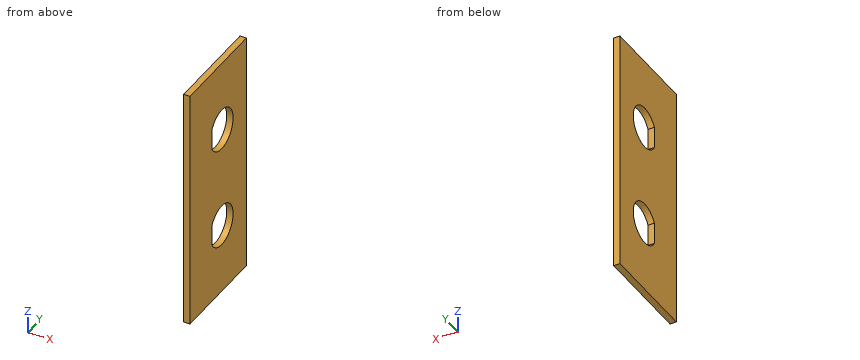
from build123d import *

# Parameters (mm, degrees)
SKETCH1_W           = 203.2
SKETCH1_H           = 120.65
BOSS_EXTRUDE1_DEPTH = 50.8
SKETCH2_W           = 196.85
SKETCH2_H           = 114.3
CUT_EXTRUDE1_DEPTH  = 51.8
SKETCH4_W           = 203.2
SKETCH4_H           = 120.65
SKETCH4_W_2         = 196.85
SKETCH4_H_2         = 114.3
BOSS_EXTRUDE2_DEPTH = 6.35
CUT_EXTRUDE5_DEPTH  = 121.65
CUT_EXTRUDE6_REACH  = 205.2
CUT_EXTRUDE7_REACH  = 205.2
SKETCH13_R          = 12.55395
SKETCH14_W          = 200.025
SKETCH14_H          = 120.65
CUT_EXTRUDE8_DEPTH  = 51.8


with BuildPart() as part:
    # Sketch1 → Boss-Extrude1 (new body)
    with BuildSketch(Plane(origin=(0, 0, 0), x_dir=(1, 0, 0), z_dir=(0, 1, 0))):
        Rectangle(SKETCH1_W, SKETCH1_H)
    extrude(amount=BOSS_EXTRUDE1_DEPTH)

    # Sketch2 → Cut-Extrude1 (cut, through all)
    with BuildSketch(Plane(origin=(0, 50.8, 0), x_dir=(1, 0, 0), z_dir=(0, 1, 0))):
        Rectangle(SKETCH2_W, SKETCH2_H)
    extrude(amount=-CUT_EXTRUDE1_DEPTH, mode=Mode.SUBTRACT)

    # Sketch4 → Boss-Extrude2 (add)
    with BuildSketch(Plane(origin=(0, 50.8, 0), x_dir=(1, 0, 0), z_dir=(0, 1, 0))):
        Rectangle(SKETCH4_W, SKETCH4_H)
        Rectangle(SKETCH4_W_2, SKETCH4_H_2, mode=Mode.SUBTRACT)
    extrude(amount=-BOSS_EXTRUDE2_DEPTH)

    # Sketch10 → Cut-Extrude5 (cut, through all)
    with BuildSketch(Plane.XY.offset(60.325)):
        with BuildLine():
            ThreePointArc((-65.9511, 22.225), (-81.206975571, 31.167602912), (-81.556705839, 13.4874))
            Line((-81.556705839, 13.4874), (-70.843294161, 13.4874))
            ThreePointArc((-70.843294161, 13.4874), (-67.257397088, 17.218024429), (-65.9511, 22.225))
        make_face()
        with BuildLine():
            ThreePointArc((-15.1511, 22.225), (-30.406975571, 31.167602912), (-30.756705839, 13.4874))
            Line((-30.756705839, 13.4874), (-20.043294161, 13.4874))
            ThreePointArc((-20.043294161, 13.4874), (-16.457397088, 17.218024429), (-15.1511, 22.225))
        make_face()
        with BuildLine():
            ThreePointArc((35.6489, 22.225), (20.393024429, 31.167602912), (20.043294161, 13.4874))
            Line((20.043294161, 13.4874), (30.756705839, 13.4874))
            ThreePointArc((30.756705839, 13.4874), (34.342602912, 17.218024429), (35.6489, 22.225))
        make_face()
        with BuildLine():
            Line((70.843294161, 13.4874), (81.556705839, 13.4874))
            ThreePointArc((81.556705839, 13.4874), (85.142602912, 17.218024429), (86.4489, 22.225))
            ThreePointArc((86.4489, 22.225), (71.193024429, 31.167602912), (70.843294161, 13.4874))
        make_face()
    extrude(amount=-CUT_EXTRUDE5_DEPTH, mode=Mode.SUBTRACT)

    # Sketch12 → Cut-Extrude6 (cut, up to next)
    with BuildSketch(Plane(origin=(101.6, 0, 0), x_dir=(0, 0, -1), z_dir=(1, 0, 0)), mode=Mode.PRIVATE) as cut_extrude6_sk1:
        with BuildLine():
            ThreePointArc((-20.043294161, 19.8374), (-25.4, 38.8239), (-30.756705839, 19.8374))
            Line((-30.756705839, 19.8374), (-20.043294161, 19.8374))
        make_face()
    cut_extrude6_tool1 = extrude(cut_extrude6_sk1.sketch, amount=-CUT_EXTRUDE6_REACH, mode=Mode.PRIVATE) & part.part
    add(cut_extrude6_tool1.solids().sort_by_distance((101.6, 28.896198, 25.4))[0], mode=Mode.SUBTRACT)
    # Sketch12 → Cut-Extrude6 (cut, up to next)
    with BuildSketch(Plane(origin=(101.6, 0, 0), x_dir=(0, 0, -1), z_dir=(1, 0, 0)), mode=Mode.PRIVATE) as cut_extrude6_sk2:
        with BuildLine():
            ThreePointArc((30.756705839, 19.8374), (25.4, 38.8239), (20.043294161, 19.8374))
            Line((20.043294161, 19.8374), (30.756705839, 19.8374))
        make_face()
    cut_extrude6_tool2 = extrude(cut_extrude6_sk2.sketch, amount=-CUT_EXTRUDE6_REACH, mode=Mode.PRIVATE) & part.part
    add(cut_extrude6_tool2.solids().sort_by_distance((101.6, 28.896198, -25.4))[0], mode=Mode.SUBTRACT)

    # Sketch13 → Cut-Extrude7 (cut, up to next)
    with BuildSketch(Plane.ZY.offset(101.6), mode=Mode.PRIVATE) as cut_extrude7_sk1:
        with Locations((15.875, 28.575)):
            Circle(SKETCH13_R)
    cut_extrude7_tool1 = extrude(cut_extrude7_sk1.sketch, amount=-CUT_EXTRUDE7_REACH, mode=Mode.PRIVATE) & part.part
    add(cut_extrude7_tool1.solids().sort_by_distance((-101.6, 28.575, 15.875))[0], mode=Mode.SUBTRACT)

    # Sketch14 → Cut-Extrude8 (cut, through all)
    with BuildSketch(Plane(origin=(0, 50.8, 0), x_dir=(1, 0, 0), z_dir=(0, 1, 0))):
        with Locations((-1.5875, 0)):
            Rectangle(SKETCH14_W, SKETCH14_H)
    extrude(amount=-CUT_EXTRUDE8_DEPTH, mode=Mode.SUBTRACT)


solid = part.part
CAD build for the part. Positions are in the model's coordinates, mm. Round coordinates to 2 decimals unless told otherwise and drop trailing zeros. Write each loop counter-clockwise with the first axis right and the second up, starting at its lowest first coordinate (ties: lowest second). Pieces come first, ordered by that corner, then holes. Notation, with made-up numbers: M 51,21 L 94,21 A13 ccw 94,36 Z; hole C -24,42.5 d4. An arc over 180 degrees is marked long. Put each result on its own line as item: value. Start each with the question number.
1) Saw through at B-B, the plane y = 28. Write the cut outline in (x, z) (3 decimals).
2) Saw through at C-C, the plane x = 100.45. Write the cut outline in (y, z) (3 decimals).
3) Saw through at A-A, the plane z = 25.4. Write the cut outline in (x, y) (3 decimals), and give its area (3 significant figures).
4) Drill centre lines: probe 1 along Z at (x, y) = (100.4, 37) (3 decimals); probe 2 along Z at (x, y) = (99.65, 21) (3 decimals); probe 3 along Y at (x, z) = (99.9, -25.4). Where is each one in solid material? Low to high. Write a range as [from, to].
5) Pin check, flat tip, straight feed: pin 1 Ø23.5 at (y, z) = (28.575, -25.4) entering from +X. Stop position of the tip, or through.
Resolved:
1. outline: M 98.425,-60.325 L 101.6,-60.325 L 101.6,-35.633 L 98.425,-35.633 Z; M 98.425,-15.167 L 101.6,-15.167 L 101.6,15.167 L 98.425,15.167 Z; M 98.425,35.633 L 101.6,35.633 L 101.6,60.325 L 98.425,60.325 Z
2. outline: M 0,-60.325 L 50.8,-60.325 L 50.8,60.325 L 0,60.325 Z; hole M 19.837,-30.757 A10.249 ccw long 19.837,-20.043 Z; hole M 19.837,20.043 A10.249 ccw long 19.837,30.757 Z
3. outline: M 98.425,0 L 101.6,0 L 101.6,19.837 L 98.425,19.837 Z; M 98.425,38.824 L 101.6,38.824 L 101.6,50.8 L 98.425,50.8 Z
3. area: 101 mm²
4. probe 1: [-60.325, -31.236], [-19.564, 19.564], [31.236, 60.325]
4. probe 2: [-60.325, -32.304], [-18.496, 18.496], [32.304, 60.325]
4. probe 3: [0, 19.84], [38.82, 50.8]
5. pin 1: x = 101.6
